```python
from build123d import *

# Parameters (mm, degrees)
SKETCH_1_R          = 4
EXTRUDE_1_DEPTH     = 9.39
SKETCH_2_R          = 3
CUT_EXTRUDE_1_DEPTH = 8
CUT_EXTRUDE_START   = -8
SKETCH_3_R          = 3
CUT_EXTRUDE_3_DEPTH = 8
SKETCH_4_R          = 8
SKETCH_4_R_2        = 4
EXTRUDE_4_DEPTH     = 2
SKETCH_5_R          = 0.99
CUT_EXTRUDE_6_DEPTH = 2


with BuildPart() as part:
    # 草图1 → 凸台-拉伸1 (new body)
    with BuildSketch(Plane.XY):
        Circle(SKETCH_1_R)
    extrude(amount=EXTRUDE_1_DEPTH)

    # 草图2 → 切除-拉伸1 (cut)
    with BuildSketch(Plane.XY.offset(9.39)):
        Circle(SKETCH_2_R)
    extrude(amount=-CUT_EXTRUDE_1_DEPTH, mode=Mode.SUBTRACT)

    # 草图3 → 切除-拉伸3 (cut)
    with BuildSketch(Plane(origin=(0, 0, 0), x_dir=(-1, 0, 0), z_dir=(0, 0, -1)).offset(CUT_EXTRUDE_START)):
        with Locations(Location((0, 0, 0), (0, 0, 180))):
            Circle(SKETCH_3_R)
    extrude(amount=CUT_EXTRUDE_3_DEPTH, mode=Mode.SUBTRACT)

    # 草图4 → 凸台-拉伸4 (add)
    with BuildSketch(Plane(origin=(0, 0, 0), x_dir=(-1, 0, 0), z_dir=(0, 0, -1))):
        Circle(SKETCH_4_R)
        Circle(SKETCH_4_R_2, mode=Mode.SUBTRACT)
    extrude(amount=-EXTRUDE_4_DEPTH)

    # 草图5 → 切除-拉伸6 (cut)
    with BuildSketch(Plane(origin=(0, 0, 0), x_dir=(-1, 0, 0), z_dir=(0, 0, -1))):
        with Locations((7, 0)):
            Circle(SKETCH_5_R)
        with Locations((4.949747468, -4.949747468)):
            Circle(SKETCH_5_R)
        with Locations((0, -7)):
            Circle(SKETCH_5_R)
        with Locations((-4.949747468, -4.949747468)):
            Circle(SKETCH_5_R)
        with Locations((-7, 0)):
            Circle(SKETCH_5_R)
        with Locations((-4.949747468, 4.949747468)):
            Circle(SKETCH_5_R)
        with Locations((0, 7)):
            Circle(SKETCH_5_R)
        with Locations((4.949747468, 4.949747468)):
            Circle(SKETCH_5_R)
    extrude(amount=-CUT_EXTRUDE_6_DEPTH, mode=Mode.SUBTRACT)


solid = part.part
```
Part model, mm, in its own coordinate system. A direction names the side the tool comes from. Give positions to 0.01 mm unless a question says otherwise; leave off trailing zeros. Write each loop counter-clockwise with the first axis right and the second up, starting at its lowest first coordinate (ties: lowest second). Pieces come first, ordered by that corner, then holes. Notation, with made-up numbers: (24, 22) -> (49, 22) arc R27 ccw to (49, 51) -> close; hole circle Ø1 at (70, 11). An arc over 180 degrees is marked (long way). Put each result on its own line as item: value. Start each with the question number.
Item 1: Cut at B-B (y = -4.25). List the corners of the cut face in (x, z).
Item 2: Which spindle directions (+Z, -Z, +X, -X, +Y, -Y) get a long thin tool onto all of the face, cutting with end or side? Do faces 1 (the face through (-0.867, -3.905, 5.643)), 2 (the face through (1, 3, 9.39)). Say none if no direction does.
Item 3: Pull direction Y, two halves, no side cores. Call faces 3 (the face through (1.73, -7.81, 0.99)), 4 (the face through (4, -2, 2)), 5 (the face through (2.86, -0.9, 4.76)): pulls with the +Y half, pulls with the -Y half, needs draft (parallel to the pull), parting line crosses it, or undercut.
Item 4: Cut at D-D (x = -5). List the corners of the cut face in (y, z) (3 decimals).
Item 5: Wall check: L1, parallel to X at y = -4.75, z = 1; L2, parallel to Z at x = -3.25, y = -5; L3, parallel to X at y = 0, z = 3. Give the ranges that are in metal, low to high. Write a range as [from, to].
Item 6: Cut at C-C (y = 0.75). List the corners of the cut face in (x, z).
Item 7: Cut at A-A (x = 0). State how many separate pieces and enclosed holes the cut face has, then the cut area to 3 significant figures.
Item 8: Pin check, flat tips, straight feed: pin 1 Ø1.8 at (x, y) = (4.95, 4.95) entering from -Z; pin 2 Ø2.5 at (x, y) = (0, 7) entering from +Z; pin 3 Ø3 at (x, z) = (0, 5) entering from +Y. Stop position of each tip, or through.
Answer list:
1. outline: (-6.78, 0) -> (-5.65, 0) -> (-5.65, 2) -> (-6.78, 2) -> close; (-4.25, 0) -> (4.25, 0) -> (4.25, 2) -> (-4.25, 2) -> close; (5.65, 0) -> (6.78, 0) -> (6.78, 2) -> (5.65, 2) -> close
2. face 1: +Z
2. face 2: +Z, +X, -X, +Y, -Y
3. face 3: parting line crosses it
3. face 4: needs draft
3. face 5: undercut
4. outline: (-6.245, 0) -> (-5.938, 0) -> (-5.938, 2) -> (-6.245, 2) -> close; (-3.961, 0) -> (3.961, 0) -> (3.961, 2) -> (-3.961, 2) -> close; (5.938, 0) -> (6.245, 0) -> (6.245, 2) -> (5.938, 2) -> close
5. L1: x = [-6.44, -5.92], [-3.98, 3.98], [5.92, 6.44]
5. L2: z = [0, 2]
5. L3: x = [-4, -3], [3, 4]
6. outline: (-7.96, 0) -> (-7.65, 0) -> (-7.65, 2) -> (-7.96, 2) -> close; (-6.35, 0) -> (-2.9, 0) -> (-2.9, 9.39) -> (-3.93, 9.39) -> (-3.93, 2) -> (-6.35, 2) -> close; (2.9, 0) -> (6.35, 0) -> (6.35, 2) -> (3.93, 2) -> (3.93, 9.39) -> (2.9, 9.39) -> close; (7.65, 0) -> (7.96, 0) -> (7.96, 2) -> (7.65, 2) -> close
7. separate pieces: 4
7. enclosed holes: 0
7. area: 26.9 mm2
8. pin 1: passes through
8. pin 2: stops at z = 2
8. pin 3: stops at y = 4
